Autodesk Inventor part; units mm, degrees
ref_plane "Work Plane2" through (0, 0, 0) normal (0, -1, 0) x (1, 0, 0)
ref_plane "Work Plane3" through (167.5, 74.771, 0) normal (0.7444, -0.6677, 0) x (0.6677, 0.7444, 0)
ref_plane "YZ Plane" through (0, 0, 0) normal (1, 0, 0) x (0, 1, 0)
sketch "Sketch1" plane through (0, 0, 0) normal (0, 0, 1) x (1, 0, 0)
  circle A0 centre (0, 225) radius 225 construction
  circle A1 centre (0, 225) radius 220 construction
  line L0 (0, 0) -> (0, 5)
  arc A2 (0, 0) -> (167.5, 74.771) centre (0, 225) ccw
  line L1 (167.5, 74.771) -> (163.7778, 78.1094)
  arc A3 (0, 5) -> (163.7778, 78.1094) centre (0, 225) ccw
  dimension "d0" = 450
  dimension "d1" = 5
  dimension "d2" = 5
  dimension "d6" = 167.5
extrude "Extrusion1" add sketch "Sketch1" along normal blind 75
ref_plane "Work Plane2" through (0, 0, 0) normal (0, -1, 0) x (1, 0, 0)
sketch "Sketch3" plane through (0, 0, 0) normal (0, -1, 0) x (1, 0, 0)
  circle A0 centre (4, 47.5) radius 3
  circle A1 centre (4, 27.5) radius 3
  point P0 (0, 0)
  dimension "d15" = 6
  dimension "d16" = 6
  dimension "d17" = 27.5
  dimension "d18" = 20
  dimension "d19" = 4
extrude "Extrusion3" cut sketch "Sketch3" along normal through all both and the other way through all
ref_plane "Work Plane3" through (167.5, 74.771, 0) normal (0.7444, -0.6677, 0) x (0.6677, 0.7444, 0)
sketch "Sketch4" plane through (167.5, 74.771, 0) normal (0.7444, -0.6677, 0) x (0.6677, 0.7444, 0)
  circle A0 centre (-55, 47.5) radius 3
  circle A1 centre (-55, 27.5) radius 3
  line L0 (-167.5, 0) -> (0, 0)
  line L1 (0, 0) -> (0, 75)
  circle A2 centre (-5, 47.5) radius 3
  circle A3 centre (-5, 27.5) radius 3
  circle A4 centre (-65, 27.5) radius 3
  circle A5 centre (-65, 47.5) radius 3
  dimension "d22" = 6
  dimension "d23" = 6
  dimension "d24" = 27.5
  dimension "d25" = 20
  dimension "d26" = 55
  dimension "d29" = 6
  dimension "d30" = 6
  dimension "d31" = 5
  dimension "d32" = 6
  dimension "d33" = 6
  dimension "d34" = 10
extrude "Extrusion4" cut sketch "Sketch4" along normal through all both and the other way through all
properties part number "CW003" material "ABS Plastic"
Could you check a few things on this model? Use its own coordinates, in mm. Coordinates: 2 decimals unless noted, no trailing zeros. Write each loop counter-clockwise with the first axis right and the second up, starting at its lowest first coordinate (ties: lowest second). Pieces come first, ordered by that corner, then holes. Notation, with made-up numbers: (89.25, 63) - (99.25, 63) arc R13 cw to (99.25, 71) - close; hole circle Ø5 at (-15, 20.25). An arc over 180 degrees is marked (long way). Write item = value, one per line.
1) Will these pins go through, and if not, where does the flat tip stop? pin 1 Ø10 at (x, z) = (46, 61) entering from -Y; pin 2 Ø2 at (x, y) = (147, 63) entering from -Z; pin 3 Ø10 at (x, z) = (133, 18.5) entering from +Y; pin 4 Ø4 at (x, z) = (55.5, 46.5) entering from -Y.
Result set:
pin_1 = 3.77
pin_2 = through
pin_3 = 53.66
pin_4 = 6.45
2) Suppose I cut it at B-B on z = 27.5. Please give me the cut outline in (x, y), plus the area to 3 significant figures.
Result set:
outline = (0, 0) arc R225 ccw to (1, 0) - (1, 5) arc R220 cw to (0, 5) - close; (7, 0.11) arc R225 ccw to (114.27, 31.17) - (110.36, 34.68) arc R220 cw to (7, 5.11) - close; (115.74, 37.91) - (119.62, 34.43) arc R225 ccw to (123.11, 36.67) - (119.26, 40.13) arc R220 cw to start; (124.42, 43.56) - (128.25, 40.13) arc R225 ccw to (162.05, 68.91) - (158.33, 72.25) arc R220 cw to start; (162.44, 76.63) - (166.16, 73.29) arc R225 ccw to (167.5, 74.77) - (163.78, 78.11) arc R220 cw to start
area = 812 mm2
3) Suppose I cut it at C-C on z = 35.5. Please give me the cut outline in (x, y).
Result set:
outline = (0, 0) arc R225 ccw to (167.5, 74.77) - (163.78, 78.11) arc R220 cw to (0, 5) - close
4) Suppose I cut it at D-D on y = 45.5. Please give me the cut outline in (x, z), plus the area to 3 significant figures.
Result set:
outline = (127.2, 0) - (135.66, 0) - (135.66, 75) - (127.2, 75) - close
area = 635 mm2
5) Please list where these lines run through material, in increasing order: line 1 (Z direction, x = 4, y = 3); line 2 (X direction, y = 30, z = 51); line 3 (Y direction, x = 74.5, z = 67). Write a range as [from, to].
Result set:
line_1 = [0, 24.5], [30.5, 44.5], [50.5, 75]
line_2 = [101.86, 112.25]
line_3 = [12.69, 18]
6) Suppose I cut it at A-A on x = 4. Please give me the cut outline in (y, z).
Result set:
outline = (0.04, 0) - (5.04, 0) - (5.04, 24.5) - (0.04, 24.5) - close; (0.04, 30.5) - (5.04, 30.5) - (5.04, 44.5) - (0.04, 44.5) - close; (0.04, 50.5) - (5.04, 50.5) - (5.04, 75) - (0.04, 75) - close
7) We'd pull the mould along X, two halves only. Please class faces 1 (the flat face through (165.66, 76.42, 36.98)), 2 (the cylindrical face through (1, 2.5, 27.6)), 3 (the flat face through (96, 25, 75)): +X half, -X half, draft (parallel to the pull), parting line (faces both ways), or undercut.
Result set:
face_1 = +X half
face_2 = undercut
face_3 = draft
